```python
from build123d import *

# Parameters (mm, degrees)
F1_DEPTH = 27.25
F2_DEPTH = 26.15
F4_T     = -1
F5_DEPTH = 3.62
F6_R     = 2


with BuildPart() as f1:
    # F0 (on Front) → F1 (new body, symmetric)
    with BuildSketch(Plane.XZ):
        Polygon((40.75, 10.1086891984), (0, 10.1086891984), (-40.75, 10.1086891984), (-40.75, 7.6086891984), (-39.75, 7.6086891984), (39.75, 7.6086891984), (40.75, 7.6086891984), align=None)
    extrude(amount=F1_DEPTH, both=True)

    # F0 (on Front) → F2 (join, symmetric)
    with BuildSketch(Plane.XZ):
        Polygon((39.75, 7.6086891984), (-39.75, 7.6086891984), (-38.3, -37.8913108016), (0, -37.8913108016), (38.3, -37.8913108016), align=None)
    extrude(amount=F2_DEPTH, both=True)

    # F4
    f4_openings = [f1.faces().sort_by_distance(p)[0] for p in [
        (0, 0, 10.108689),
    ]]
    offset(amount=F4_T, openings=f4_openings, kind=Kind.INTERSECTION)

    # F3 (on face) → F5 (join)
    with BuildSketch(Plane(origin=(0, 0, -37.8913108016), x_dir=(1, 0, 0), z_dir=(0, 0, -1))):
        with BuildLine():
            ThreePointArc((-38.3, 23.9), (-36.05, 21.65), (-33.8, 23.9))
            ThreePointArc((-33.8, 23.9), (-34.4590097351, 25.4909902504), (-36.0499999795, 26.15))
            ThreePointArc((-36.0499999795, 26.15), (-37.6409902504, 25.4909902649), (-38.3, 23.9))
        make_face()
        with BuildLine():
            ThreePointArc((-33.8, -23.9), (-36.0499999898, -21.65), (-38.3, -23.8999999795))
            ThreePointArc((-38.3, -23.8999999795), (-37.6409902649, -25.4909902504), (-36.05, -26.15))
            ThreePointArc((-36.05, -26.15), (-34.4590097423, -25.4909902577), (-33.8, -23.9))
        make_face()
        with BuildLine():
            ThreePointArc((36.05, -26.15), (37.6409902577, -25.4909902577), (38.3, -23.9))
            ThreePointArc((38.3, -23.9), (34.4590097423, -22.3090097423), (36.05, -26.15))
        make_face()
        with BuildLine():
            ThreePointArc((38.3, 23.9), (37.6409902577, 25.4909902577), (36.05, 26.15))
            ThreePointArc((36.05, 26.15), (34.4590097423, 22.3090097423), (38.3, 23.9))
        make_face()
    extrude(amount=F5_DEPTH)

    # F6
    f6_edges = [f1.edges().sort_by_distance(p)[0] for p in [
        (-39.025, -26.15, -15.141311),
        (39.025, -26.15, -15.141311),
        (39.025, 26.15, -15.141311),
        (-39.025, 26.15, -15.141311),
        (-40.75, 27.25, 8.858689),
        (-40.75, -27.25, 8.858689),
        (40.75, -27.25, 8.858689),
        (40.75, 27.25, 8.858689),
        (38.05636, -25.15, -14.141311),
        (-38.05636, -25.15, -14.141311),
        (-38.05636, 25.15, -14.141311),
        (38.05636, 25.15, -14.141311),
        (39.75, 26.25, 9.358689),
        (-39.75, 26.25, 9.358689),
        (39.75, -26.25, 9.358689),
        (-39.75, -26.25, 9.358689),
    ]]
    fillet(f6_edges, radius=F6_R)


solid = f1.part
```
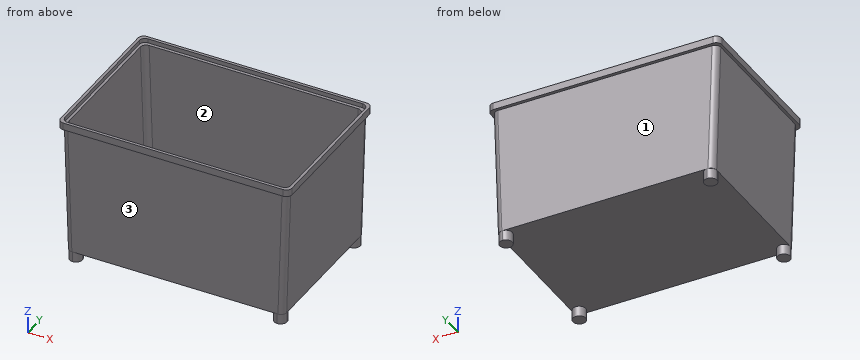
Geometry check sheet. Reference: the model listing, model coordinates, mm. Face numbers are marked on the shaded views. Coordinates: 2 decimals unless noted, no trailing zeros. Write each loop counter-clockwise with the first axis right and the second up, starting at its lowest first coordinate (ties: lowest second). Pieces come first, ordered by that corner, then holes. Notation, with made-up numbers: (38.5, 34.25) -> (45.5, 34.25) arc R20 ccw to (45.5, 63.25) -> close; hole circle Ø2 at (55, -13). An arc over 180 degrees is marked (long way). Use CSV: the item, a comma, the result in double quotes. Start each with the question number.
Item 1: Depth check by flat-ended pin: pin 1 Ø5 at (y, z) = (16.5, -5) entering from +X; pin 2 Ø4 at (x, z) = (-10, -22.5) entering from +Y; pin 3 Ø1 at (y, z) = (-10, -2) entering from -X. Enter the tip coordinate at first touch or a pass-through.
Item 2: Cross-section at B-B, the plane y = 3. Record the cut outline in (x, z), plus the area to 3 significant figures.
Item 3: Thickness scan on line 1 (X direction, y = -5.5, z = 7); line 2 (Y direction, x = 22, z = -34); line 3 (X direction, y = -15.5, z = -23.5). Record the ranges inside material, lowest first.
Item 4: Mould release check, pull along Y, two halves, no side actions. Record for the marked faces 1, 2 and 3: released by +Y, released by -Y, zero draft, split by the parting line, or undercut.
Item 5: Cross-section at A-A, the plane x = -13. Record the cut outline in (y, z).
Answers:
1,pin 1,"x = 39.43"
1,pin 2,"y = 26.15"
1,pin 3,"x = -39.46"
2,outline,"(-40.75, 7.61) -> (-39.75, 7.61) -> (-38.3, -37.89) -> (38.3, -37.89) -> (39.75, 7.61) -> (40.75, 7.61) -> (40.75, 10.11) -> (39.75, 10.11) -> (39.75, 8.61) -> (38.78, 8.61) -> (37.33, -36.89) -> (-37.33, -36.89) -> (-38.78, 8.61) -> (-39.75, 8.61) -> (-39.75, 10.11) -> (-40.75, 10.11) -> close"
2,area,"173 mm^2"
3,line 1,"-39.73 to -38.73, 38.73 to 39.73"
3,line 2,"-26.15 to -25.15, 25.15 to 26.15"
3,line 3,"-38.76 to -37.76, 37.76 to 38.76"
4,face 1,"released by +Y"
4,face 2,"undercut"
4,face 3,"released by -Y"
5,outline,"(-27.25, 7.61) -> (-26.15, 7.61) -> (-26.15, -37.89) -> (26.15, -37.89) -> (26.15, 7.61) -> (27.25, 7.61) -> (27.25, 10.11) -> (26.25, 10.11) -> (26.25, 8.61) -> (25.15, 8.61) -> (25.15, -36.89) -> (-25.15, -36.89) -> (-25.15, 8.61) -> (-26.25, 8.61) -> (-26.25, 10.11) -> (-27.25, 10.11) -> close"
